Source: CAD feature listing. Evaluate the final solid. Frame: model axes, mm. Give positions to 0.01 mm unless a question says otherwise; leave off trailing zeros. Write each loop counter-clockwise with the first axis right and the second up, starting at its lowest first coordinate (ties: lowest second). Pieces come first, ordered by that corner, then holes. Notation, with made-up numbers: (-15, 21.25) -> (8, 21.25) arc R13 cw to (8, 29.25) -> close; hole circle Ø11 at (-28, 34). An arc over 180 degrees is marked (long way). Answer as a JSON object with one key per item and string values. Group by question number.
Item 1: First-contact query: pin 1 Ø1 at (y, z) = (2, -25) entering from -X; pin 2 Ø1.6 at (y, z) = (2, -25.5) entering from +X. Flat tips, straight axial feed; report the tip coordinate or a pass-through.
Item 2: Ray query, probe 1 along X at (y, z) = (0.75, -31); probe 2 along Z at (x, y) = (14, 0.5); probe 3 along X at (y, z) = (1.6, -22). Return the intervals inside material, ascending. Write a range as from..to.
Item 3: Section query A-A on z = -29. Return the cut outline in (x, y) (1 decimal).
Item 4: Section query C-C on z = -25. Return the cut outline in (x, y) (3 decimals).
Item 5: Section query B-B on y = 0.5. Return the cut outline in (x, z).
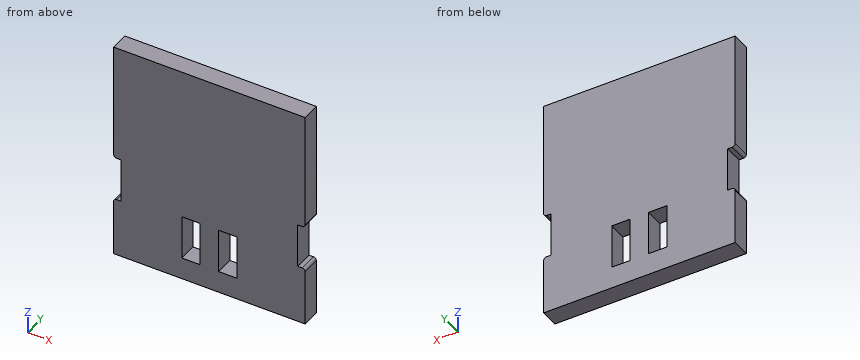
from build123d import *

# Parameters (mm, degrees)
SKETCH1_W           = 33.02
SKETCH1_H           = 38.1
SKETCH1_W_2         = 3.175
SKETCH1_H_2         = 7.62
BOSS_EXTRUDE1_DEPTH = 3.175
SKETCH5_W           = 1.27
SKETCH5_H           = 7.62
CUT_EXTRUDE3_DEPTH  = 51.517432882
FILLET2_R           = 0.508


with BuildPart() as part:
    # Sketch1 → Boss-Extrude1 (new body)
    with BuildSketch(Plane(origin=(0, 0, 0), x_dir=(1, 0, 0), z_dir=(0, 1, 0))):
        with Locations((16.51, 19.05)):
            Rectangle(SKETCH1_W, SKETCH1_H)
        with Locations((13.335, 30.48)):
            Rectangle(SKETCH1_W_2, SKETCH1_H_2, mode=Mode.SUBTRACT)
        with Locations((19.685, 30.48)):
            Rectangle(SKETCH1_W_2, SKETCH1_H_2, mode=Mode.SUBTRACT)
    extrude(amount=BOSS_EXTRUDE1_DEPTH)

    # Sketch5 → Cut-Extrude3 (cut, through all)
    with BuildSketch(Plane.XZ):
        with Locations((32.385, -24.13)):
            Rectangle(SKETCH5_W, SKETCH5_H)
        with Locations((0.635, -24.13)):
            Rectangle(SKETCH5_W, SKETCH5_H)
    extrude(amount=-CUT_EXTRUDE3_DEPTH, mode=Mode.SUBTRACT)

    # Fillet2
    fillet2_edges = [part.edges().sort_by_distance(p)[0] for p in [
        (33.02, 1.5875, -20.32),
        (33.02, 1.5875, -27.94),
        (0, 1.5875, -27.94),
        (0, 1.5875, -20.32),
    ]]
    fillet(fillet2_edges, radius=FILLET2_R)


solid = part.part
Worked answers:
{
 "1": {"pin 1": "x = 1.27", "pin 2": "x = 31.75"},
 "2": {"probe 1": "0..11.75, 14.92..18.1, 21.27..33.02", "probe 2": "-38.1..-34.29, -26.67..0", "probe 3": "1.27..31.75"},
 "3": {"outline": "(0, 0) -> (11.7, 0) -> (11.7, 3.2) -> (0, 3.2) -> close; (14.9, 0) -> (18.1, 0) -> (18.1, 3.2) -> (14.9, 3.2) -> close; (21.3, 0) -> (33, 0) -> (33, 3.2) -> (21.3, 3.2) -> close"},
 "4": {"outline": "(1.27, 0) -> (31.75, 0) -> (31.75, 3.175) -> (1.27, 3.175) -> close"},
 "5": {"outline": "(0, -38.1) -> (33.02, -38.1) -> (33.02, -28.45) arc R0.51 ccw to (32.51, -27.94) -> (31.75, -27.94) -> (31.75, -20.32) -> (32.51, -20.32) arc R0.51 ccw to (33.02, -19.81) -> (33.02, 0) -> (0, 0) -> (0, -19.81) arc R0.51 ccw to (0.51, -20.32) -> (1.27, -20.32) -> (1.27, -27.94) -> (0.51, -27.94) arc R0.51 ccw to (0, -28.45) -> close; hole (11.75, -34.29) -> (14.92, -34.29) -> (14.92, -26.67) -> (11.75, -26.67) -> close; hole (18.1, -34.29) -> (21.27, -34.29) -> (21.27, -26.67) -> (18.1, -26.67) -> close"}
}
